from build123d import *

# Parameters (mm, degrees)
SKETCH1_R           = 35
BOSS_EXTRUDE1_DEPTH = 2
SKETCH2_R           = 5
CUT_EXTRUDE2_DEPTH  = 2
SKETCH4_R           = 8
SKETCH4_R_2         = 5
BOSS_EXTRUDE3_DEPTH = 10
FILLET3_R           = 0.75
FILLET4_R           = 1.5
BOSS_EXTRUDE4_START = 0.2
BOSS_EXTRUDE4_DEPTH = 2.5
BOSS_EXTRUDE5_START = 2.7
BOSS_EXTRUDE5_DEPTH = 2.5
SKETCH7_R           = 1.25
CUT_EXTRUDE3_DEPTH  = 60.240948676


with BuildPart() as part:
    # Sketch1 → Boss-Extrude1 (new body)
    with BuildSketch(Plane.XY):
        Circle(SKETCH1_R)
    extrude(amount=BOSS_EXTRUDE1_DEPTH)

    # Sketch2 → Cut-Extrude2 (cut)
    with BuildSketch(Plane.XY.offset(2)):
        with Locations((0, 25)):
            Circle(SKETCH2_R)
    extrude(amount=-CUT_EXTRUDE2_DEPTH, mode=Mode.SUBTRACT)

    # Sketch4 → Boss-Extrude3 (add)
    with BuildSketch(Plane(origin=(0, 0, 0), x_dir=(-1, 0, 0), z_dir=(0, 0, -1))):
        with Locations(Location((0, 25, 0), (0, 0, 180))):
            Circle(SKETCH4_R)
        with Locations(Location((0, 25, 0), (0, 0, 180))):
            Circle(SKETCH4_R_2, mode=Mode.SUBTRACT)
    extrude(amount=BOSS_EXTRUDE3_DEPTH)

    # Fillet3
    fillet3_edges = [part.edges().sort_by_distance(p)[0] for p in [
        (-5, 25, -10),
    ]]
    fillet(fillet3_edges, radius=FILLET3_R)

    # Fillet4
    fillet4_edges = [part.edges().sort_by_distance(p)[0] for p in [
        (-8, 25, -10),
    ]]
    fillet(fillet4_edges, radius=FILLET4_R)

    # Sketch5 → Boss-Extrude4 (add)
    with BuildSketch(Plane(origin=(8, 0, 0), x_dir=(0, 0, -1), z_dir=(1, 0, 0)).offset(BOSS_EXTRUDE4_START)):
        with BuildLine():
            Line((13, 15.769174864), (0, 15.769174864))
            Line((0, 15.769174864), (0, 11.769174864))
            Line((0, 11.769174864), (10, 11.769174864))
            ThreePointArc((10, 11.769174864), (13.5, 12.269174864), (13, 15.769174864))
        make_face()
    extrude(amount=BOSS_EXTRUDE4_DEPTH)

    # Sketch6 → Boss-Extrude5 (add)
    with BuildSketch(Plane.ZY.offset(8).offset(BOSS_EXTRUDE5_START)):
        with BuildLine():
            Line((-10, 11.769174864), (0, 11.769174864))
            Line((0, 11.769174864), (0, 15.769174864))
            Line((0, 15.769174864), (-13, 15.769174864))
            ThreePointArc((-13, 15.769174864), (-13.5, 12.269174864), (-10, 11.769174864))
        make_face()
    extrude(amount=-BOSS_EXTRUDE5_DEPTH)

    # Sketch7 → Cut-Extrude3 (cut, through all)
    with BuildSketch(Plane.ZY.offset(10.7)):
        with Locations(Location((-11.5, 13.769174864, 0), (0, 0, 270))):
            Circle(SKETCH7_R)
    extrude(amount=-CUT_EXTRUDE3_DEPTH, mode=Mode.SUBTRACT)


solid = part.part
Work out the finished part from the listing and answer in its coordinate system (mm). A direction names the side the tool comes from. Round coordinates to 2 decimals unless told otherwise and drop trailing zeros. Loops run counter-clockwise (first coordinate to the right, second up) from the corner with the lowest first, then second, coordinate; pieces in that order, holes last. Notation, with made-up numbers: (56, 64) -> (87, 64) arc R24 ccw to (87, 95) -> close; hole circle Ø4 at (80, 60.25). An arc over 180 degrees is marked (long way). Use one line per item in the form item = value.
(1) Flat-ended cylindrical pins translate along their axes: P1, Ø4, axis at y = 13.77, z = -11.5, coming from the +X side; P2, Ø9, axis at x = 0, y = 25, coming from the +Z side; P3, Ø3, axis at x = -9.5, z = -2.5, coming from the -Y side; P4, Ø8, axis at y = -20.5, z = -3, coming from the -X side. Find the tip coordinate at first contact, or state that the pin passes through.
Answer list:
P1 = 10.7
P2 = through
P3 = 11.77
P4 = -30.1
(2) Find section B-B on x = 0. Give the vertices of the cut face in (y, z), then the cut area to 3 significant figures.
Answer list:
outline = (-35, 0) -> (17, 0) -> (17, -8.5) arc R1.5 ccw to (18.5, -10) -> (19.25, -10) arc R0.75 ccw to (20, -9.25) -> (20, 2) -> (-35, 2) -> close; (30, -9.25) arc R0.75 ccw to (30.75, -10) -> (31.5, -10) arc R1.5 ccw to (33, -8.5) -> (33, 0) -> (35, 0) -> (35, 2) -> (30, 2) -> close
area = 179 mm2
(3) For a pull along Y with two mould halves and no side action, classify faces 6 (the cylindrical face through (-9.468, 13.097, -10.446)), 7 (the flat face through (9, 11.769, -5)), 8 (the cylindrical face through (9.433, 13.097, -10.446)), 9 (the flat face through (8.2, 14, -7)) as released by +Y, released by -Y, zero draft, split by the parting line, or undercut.
Answer list:
face_6 = undercut
face_7 = released by -Y
face_8 = undercut
face_9 = zero draft
(4) Find section C-C on y = 25. Give the vertices of the cut face in (x, z).
Answer list:
outline = (-24.49, 0) -> (-8, 0) -> (-8, -8.5) arc R1.5 ccw to (-6.5, -10) -> (-5.75, -10) arc R0.75 ccw to (-5, -9.25) -> (-5, 2) -> (-24.49, 2) -> close; (5, -9.25) arc R0.75 ccw to (5.75, -10) -> (6.5, -10) arc R1.5 ccw to (8, -8.5) -> (8, 0) -> (24.49, 0) -> (24.49, 2) -> (5, 2) -> close
(5) Straight lines are drawn through the part: line 1 (Y direction, x = 0, z = 1); line 2 (Y direction, x = 0, z = -2); line 3 (X direction, y = 25, z = -6.75). For each, find the intervals that lie inside material, in ascending order.
Answer list:
line_1 = -35 to 20, 30 to 35
line_2 = 17 to 20, 30 to 33
line_3 = -8 to -5, 5 to 8
(6) Find section A-A on z = -6.5. Give the vertices of the cut face in (x, y), then the cut area to 3 significant figures.
Answer list:
outline = (-10.7, 11.77) -> (-8.2, 11.77) -> (-8.2, 15.77) -> (-10.7, 15.77) -> close; circle Ø16 at (0, 25); (8.2, 11.77) -> (10.7, 11.77) -> (10.7, 15.77) -> (8.2, 15.77) -> close; hole circle Ø10 at (0, 25)
area = 143 mm2
(7) Find section D-D on z = -11.5. Give the vertices of the cut face in (x, y), then the cut area to 3 significant figures.
Answer list:
outline = (-10.7, 11.27) -> (-8.2, 11.27) -> (-8.2, 12.52) -> (-10.7, 12.52) -> close; (-10.7, 15.02) -> (-8.2, 15.02) -> (-8.2, 15.77) -> (-10.7, 15.77) -> close; (8.2, 11.27) -> (10.7, 11.27) -> (10.7, 12.52) -> (8.2, 12.52) -> close; (8.2, 15.02) -> (10.7, 15.02) -> (10.7, 15.77) -> (8.2, 15.77) -> close
area = 10.0 mm2
(8) A tool of negligible diameter and unlimited length cuts with its end or side. For faces 1 (the flat face through (10.7, 14, -7)), 2 (the cylindrical face through (-1.73, 32.81, -4.19)), 3 (the flat face through (-9, 11.769, -5)), 4 (the flat face through (9, 15.769, -7)), 5 (the flat face through (-10.7, 14, -7)), from which of +Z, -Z, +X, -X, +Y, -Y can it reach the whole face along a straight path? Write none if from no direction.
Answer list:
face_1 = -Z, +X, +Y, -Y
face_2 = -Z
face_3 = +X, -X, -Y
face_4 = -Z, +X, -X, +Y
face_5 = -Z, -X, +Y, -Y
